```python
from build123d import *

# Parameters (mm, degrees)
SKETCH_2_R          = 1.5
EXTRUDE_1_DEPTH     = 83
SKETCH_3_W          = 62.5
SKETCH_3_H          = 1
SKETCH_3_W_2        = 4.5
SKETCH_3_W_3        = 67
EXTRUDE_2_DEPTH     = 7
CUT_EXTRUDE_1_DEPTH = 83
SKETCH_5_W          = 6.8
SKETCH_5_H          = 16.9
CUT_EXTRUDE_2_DEPTH = 79
SKETCH_7_W          = 6.8
SKETCH_7_H          = 7
EXTRUDE_3_DEPTH     = 38.5
SKETCH_8_W          = 6.8
SKETCH_8_H          = 7
CUT_EXTRUDE_3_DEPTH = 32
SKETCH_9_W          = 5.5
SKETCH_9_H          = 2.7
CUT_EXTRUDE_4_DEPTH = 7


with BuildPart() as part:
    # Эскиз2 → Бобышка-Вытянуть1 (new body)
    with BuildSketch(Plane.XY):
        with BuildLine():
            Line((29, 14.5), (32.5, 21.5))
            Line((32.5, 21.5), (33.5, 21.5))
            Line((33.5, 21.5), (29.5, 13.5))
            Line((29.5, 13.5), (3.4, 13.5))
            Line((3.4, 13.5), (3.4, 0))
            ThreePointArc((3.4, 0), (0, -3.4), (-3.4, 0))
            Line((-3.4, 0), (-3.4, 13.5))
            Line((-3.4, 13.5), (-33.5, 13.5))
            Line((-33.5, 13.5), (-33.5, 14.5))
            Line((-33.5, 14.5), (-32.5, 14.5))
            Line((-32.5, 14.5), (29, 14.5))
        make_face()
        Circle(SKETCH_2_R, mode=Mode.SUBTRACT)
    extrude(amount=EXTRUDE_1_DEPTH)

    # Эскиз3 → Бобышка-Вытянуть2 (add)
    with BuildSketch(Plane(origin=(0, 14.5, 0), x_dir=(1, 0, 0), z_dir=(0, 1, 0))):
        with Locations((-2.25, -82.5)):
            Rectangle(SKETCH_3_W, SKETCH_3_H)
        with Locations((31.25, -82.5)):
            Rectangle(SKETCH_3_W_2, SKETCH_3_H)
        with Locations((0, -0.5)):
            Rectangle(SKETCH_3_W_3, SKETCH_3_H)
    extrude(amount=EXTRUDE_2_DEPTH)

    # Эскиз4 → Вырез-Вытянуть1 (cut)
    with BuildSketch(Plane.XY.offset(83)):
        Polygon((29.5, 13.5), (33.5, 21.5), (33.5, 14.5), align=None)
    extrude(amount=-CUT_EXTRUDE_1_DEPTH, mode=Mode.SUBTRACT)

    # Эскиз5 → Вырез-Вытянуть2 (cut)
    with BuildSketch(Plane.XY.offset(83)):
        with Locations((0, 5.05)):
            Rectangle(SKETCH_5_W, SKETCH_5_H)
    extrude(amount=-CUT_EXTRUDE_2_DEPTH, mode=Mode.SUBTRACT)

    # Эскиз7 → Бобышка-Вытянуть3 (add)
    with BuildSketch(Plane.XY.offset(83)):
        with Locations((0, 10)):
            Rectangle(SKETCH_7_W, SKETCH_7_H)
    extrude(amount=-EXTRUDE_3_DEPTH)

    # Эскиз8 → Вырез-Вытянуть3 (cut)
    with BuildSketch(Plane.XY.offset(83)):
        with Locations((0, 10)):
            Rectangle(SKETCH_8_W, SKETCH_8_H)
    extrude(amount=-CUT_EXTRUDE_3_DEPTH, mode=Mode.SUBTRACT)

    # Эскиз9 → Вырез-Вытянуть4 (cut)
    with BuildSketch(Plane.XZ.offset(-6.5)):
        with Locations((0, 47.75)):
            Rectangle(SKETCH_9_W, SKETCH_9_H)
    extrude(amount=-CUT_EXTRUDE_4_DEPTH, mode=Mode.SUBTRACT)


solid = part.part
```
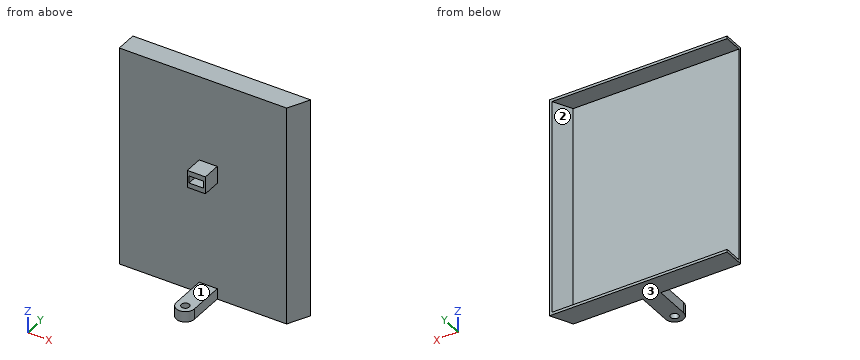
Geometry check sheet. Reference: the model listing, model coordinates, mm. Face numbers are marked on the shaded views. A direction names the side the tool comes from. Round coordinates to 2 decimals unless told otherwise and drop trailing zeros. Loops run counter-clockwise (first coordinate to the right, second up) from the corner with the lowest first, then second, coordinate; pieces in that order, holes last. Notation, with made-up numbers: (1.25, -4) -> (7.25, -4) arc R13 cw to (7.25, 15) -> close; hole circle Ø9 at (69, -24). An arc over 180 degrees is marked (long way). Use a Markdown table: item, result.
(1) Sectioned sample at C-C (y = 18). Enter the section's corners in (x, z), then the cut area to 4 significant figures.
Calculated:
| item | result |
|---|---|
| outline | (-33.5, 0) -> (31.75, 0) -> (31.75, 83) -> (-33.5, 83) -> (-33.5, 82) -> (30.75, 82) -> (30.75, 1) -> (-33.5, 1) -> close |
| area | 211.5 mm² |
(2) Go/stop test with flat-tipped pins: P1, Ø4.5, axis at y = 6.5, z = 1, coming from the +X side; P2, Ø5, axis at x = 0, z = 48, coming from the -Y side; P3, Ø0.8, axis at x = 1, z = 47, coming from the -Y side; P4, Ø8, axis at y = 0, z = 10, coming from the -X side. Record where each tip stops, or that it passes through.
Calculated:
| item | result |
|---|---|
| P1 | x = 3.4 |
| P2 | y = 6.5 |
| P3 | y = 13.5 |
| P4 | through |
(3) Sectioned sample at A-A (y = 11.75). Enter the section's corners in (x, z), then the cut area to 4 significant figures.
Calculated:
| item | result |
|---|---|
| outline | (-3.4, 0) -> (3.4, 0) -> (3.4, 4) -> (-3.4, 4) -> close; (-3.4, 44.5) -> (3.4, 44.5) -> (3.4, 51) -> (-3.4, 51) -> close; hole (-2.75, 46.4) -> (2.75, 46.4) -> (2.75, 49.1) -> (-2.75, 49.1) -> close |
| area | 56.55 mm² |
(4) Sectioned sample at D-D (x = -28). Enter the section's corners in (y, z).
Calculated:
| item | result |
|---|---|
| outline | (13.5, 0) -> (21.5, 0) -> (21.5, 1) -> (14.5, 1) -> (14.5, 82) -> (21.5, 82) -> (21.5, 83) -> (13.5, 83) -> close |
(5) Sectioned sample at B-B (x = 0). Enter the section's corners in (y, z), then the cut area to 3 significant figures.
Calculated:
| item | result |
|---|---|
| outline | (-3.4, 0) -> (-1.5, 0) -> (-1.5, 4) -> (-3.4, 4) -> close; (1.5, 0) -> (21.5, 0) -> (21.5, 1) -> (14.5, 1) -> (14.5, 82) -> (21.5, 82) -> (21.5, 83) -> (13.5, 83) -> (13.5, 51) -> (6.5, 51) -> (6.5, 49.1) -> (13.5, 49.1) -> (13.5, 46.4) -> (6.5, 46.4) -> (6.5, 44.5) -> (13.5, 44.5) -> (13.5, 4) -> (1.5, 4) -> close |
| area | 179 mm² |
(6) Set-up check for the marked faces 1, 2 and 3: record each of +Z, -Z, +X, -X, +Y, -Y from which the full face is reachable in a straight line by a thin tool's end or side.
Calculated:
| item | result |
|---|---|
| face 1 | +X, -X, -Y |
| face 2 | -X, +Y |
| face 3 | -Z, +X, -X, +Y, -Y |
(7) Scan lines: probe 1 along Z at (x, y) = (20, 20.5); probe 2 along Z at (x, y) = (-3, 7); probe 3 along Y at (x, z) = (0, 1.9). Record each from-to range of solid material in increasing order.
Calculated:
| item | result |
|---|---|
| probe 1 | 0 to 1, 82 to 83 |
| probe 2 | 0 to 4, 44.5 to 51 |
| probe 3 | -3.4 to -1.5, 1.5 to 14.5 |
